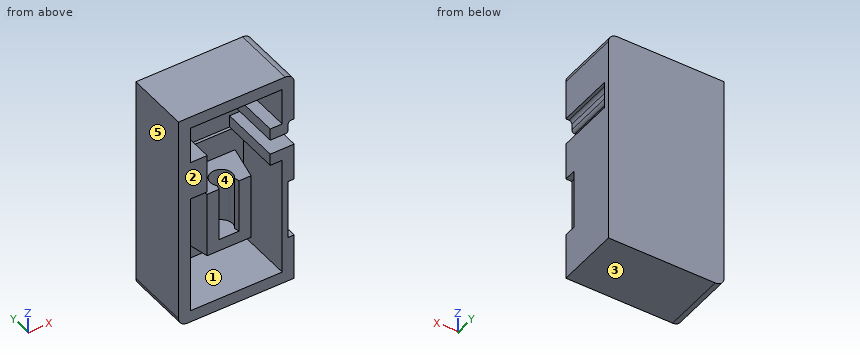
Autodesk Inventor part; units mm, degrees
ref_plane "YZ Plane" through (0, 0, 0) normal (1, 0, 0) x (0, 1, 0)
ref_plane "XZ Plane" through (0, 0, 0) normal (0, 1, 0) x (-1, 0, 0)
ref_plane "XY Plane" through (0, 0, 0) normal (0, 0, 1) x (1, 0, 0)
sketch "Sketch1" plane through (0, 0, 0) normal (0, 1, 0) x (-1, 0, 0)
  line L0 (0, 0) -> (24.5364, 0)
  line L1 (24.5364, 0) -> (24.5364, -46.5582)
  line L2 (24.5364, -46.5582) -> (0, -46.5582)
  line L3 (0, -46.5582) -> (0, 0)
  dimension "d0" = 46.5582
  dimension "d1" = 24.5364
extrude "Extrusion1" add sketch "Sketch1" along normal blind 13.5382
sketch "Sketch2" plane through (0, 0, 0) normal (0, -1, 0) x (1, 0, 0)
  point P0 (0, 0)
fillet "Fillet1" radius 1.905 1 edges at (-24.5364, 6.7691, -46.5582)
fillet "Fillet2" radius 1.905 1 edges at (0, 6.7691, 0)
sketch "Sketch3" plane through (0, 0, 0) normal (0, -1, 0) x (1, 0, 0)
  line L0 (-1.905, 0) -> (-24.5364, 0)
  arc A0 (0, -1.905) -> (-1.905, 0) centre (-1.905, -1.905) ccw
  line L1 (0, -46.5582) -> (0, -1.905)
  line L2 (-22.6314, -46.5582) -> (0, -46.5582)
  arc A1 (-24.5364, -44.6532) -> (-22.6314, -46.5582) centre (-22.6314, -44.6532) ccw
  line L3 (-24.5364, 0) -> (-24.5364, -44.6532)
  line L4 (-2.54, -2.54) -> (-21.9964, -2.54)
  line L5 (-21.9964, -44.0182) -> (-2.54, -44.0182)
  line L6 (0, -12.9032) -> (-5.08, -12.9032)
  line L7 (-5.08, -16.0782) -> (0, -16.0782)
  line L8 (-2.54, -44.0182) -> (-2.54, -18.6182)
  line L9 (-2.54, -10.3632) -> (-2.54, -2.54)
  line L10 (-5.08, -12.9032) -> (-5.08, -10.3632)
  line L11 (-5.08, -10.3632) -> (-2.54, -10.3632)
  line L12 (-5.08, -16.0782) -> (-5.08, -18.6182)
  line L13 (-5.08, -18.6182) -> (-2.54, -18.6182)
  line L14 (-21.9964, -10.3632) -> (-18.4404, -10.3632)
  line L15 (-18.4404, -10.3632) -> (-18.4404, -18.6182)
  line L16 (-18.4404, -18.6182) -> (-21.9964, -18.6182)
  line L17 (-21.9964, -2.54) -> (-21.9964, -10.3632)
  line L18 (-21.9964, -18.6182) -> (-21.9964, -44.0182)
  line L19 (0, -14.4907) -> (-5.2569, -14.4907) construction
  line L20 (-5.08, -11.6332) -> (-18.4404, -11.6332)
  line L21 (-5.08, -17.3482) -> (-18.4404, -17.3482)
  point P0 (0, 0)
  dimension "d7" = 2.54
  dimension "d9" = 2.54
  dimension "d11" = 3.175
  dimension "d13" = 5.08
  dimension "d14" = 2.54
  dimension "d15" = 2.54
  dimension "d16" = 2.54
  dimension "d17" = 2.54
  dimension "d20" = 2.54
  dimension "d21" = 6.096
  dimension "d22" = 2.54
  dimension "d37" = 32.0675
extrude "Extrusion2" cut sketch "Sketch3" against normal blind 12.2682 contours L1 L7 L12 L21 L15 L20 L10 L6 | L20 L15 L14 L17 L4 L9 L11 L10 | L12 L13 L8 L5 L18 L16 L15 L21
sketch "Sketch4" plane through (0, 12.2682, 0) normal (0, -1, 0) x (1, 0, 0)
  line L0 (-4.3434, -23.6982) -> (-17.0434, -23.6982)
  line L1 (-17.0434, -23.6982) -> (-17.0434, -35.1282)
  line L2 (-17.0434, -35.1282) -> (-4.3434, -35.1282)
  line L3 (-4.3434, -35.1282) -> (-4.3434, -23.6982)
  line L4 (-2.54, -44.0182) -> (-21.9964, -44.0182)
  line L5 (-2.54, -18.6182) -> (-2.54, -44.0182)
  line L6 (-10.6934, -23.6982) -> (-10.6934, -35.1282) construction
  line L7 (-24.5364, 0) -> (-24.5364, -44.6532) construction
  line L8 (-22.6314, -46.5582) -> (0, -46.5582) construction
  point P0 (0, 0)
  dimension "d23" = 13.843
  dimension "d24" = 12.7
  dimension "d25" = 11.43
  dimension "d26" = 22.86
extrude "Extrusion3" add sketch "Sketch4" along normal up to surface (12.2682 mm away)
sketch "Sketch5" plane through (-4.3434, 12.2682, -35.1282) normal (0, 0, -1) x (-1, 0, 0)
  line L0 (0, 0) -> (0, -12.2682)
  line L1 (12.7, 0) -> (12.7, -12.2682)
  line L2 (12.7, -12.2682) -> (0, -12.2682)
  arc A0 (8.2396, -6.5778) -> (4.4604, -6.5778) centre (6.35, -5.1816) ccw
  line L3 (6.35, -12.2682) -> (6.35, 0) construction
  line L4 (17.653, 0) -> (-1.8034, 0) construction
  line L5 (8.2396, -6.5778) -> (8.4707, -7.62)
  line L6 (8.4707, -7.62) -> (11.0107, -7.62)
  line L7 (11.0107, -7.62) -> (12.7, 0)
  line L8 (4.4604, -6.5778) -> (4.2293, -7.62)
  line L9 (4.2293, -7.62) -> (1.6893, -7.62)
  line L10 (1.6893, -7.62) -> (0, 0)
  point P0 (-4.3434, -12.2682)
  dimension "d29" = 7.0866
  dimension "d30" = 4.699
  dimension "d32" = 7.62
  dimension "d33" = 2.54
  dimension "d36" = 25
extrude "Extrusion4" cut sketch "Sketch5" against normal up to surface (11.43 mm away)
sketch "Sketch6" plane through (0, 12.2682, 0) normal (0, -1, 0) x (1, 0, 0)
  line L0 (-5.08, -10.3632) -> (-5.08, -12.9032)
  line L1 (-5.08, -16.0782) -> (-5.08, -18.6182)
  line L2 (-18.4404, -18.6182) -> (-18.4404, -10.3632)
  line L3 (0, -12.9032) -> (0, -16.0782)
  line L4 (0, -16.0782) -> (-5.08, -16.0782)
  line L5 (-5.08, -12.9032) -> (0, -12.9032)
  line L6 (-5.08, -10.3632) -> (-18.4404, -10.3632)
  line L7 (-18.4404, -18.6182) -> (-5.08, -18.6182)
  line L8 (-1.27, -12.9032) -> (-1.27, -16.0782)
  point P0 (0, 0)
  dimension "d46" = 1.27
extrude "Extrusion5" cut sketch "Sketch6" against normal blind 0.635
sketch "Sketch7" plane through (0, 0, 0) normal (0, -1, 0) x (1, 0, 0)
  line L0 (0, -12.9032) -> (0, -1.905)
  line L1 (0, -1.905) -> (0, -46.5582)
  line L2 (0, -10.3632) -> (-0.635, -10.3632)
  line L3 (-1.27, -10.9982) -> (-1.27, -12.2682)
  arc A0 (-0.635, -10.3632) -> (-1.27, -10.9982) centre (-0.635, -10.9982) ccw
  line L4 (-1.905, -12.9032) -> (-5.08, -12.9032)
  line L5 (-5.08, -10.3632) -> (-5.08, -12.9032)
  arc A1 (-1.905, -12.9032) -> (-1.27, -12.2682) centre (-1.905, -12.2682) ccw
  line L6 (0, -10.3632) -> (0, -12.9032)
  line L7 (0, -12.9032) -> (-1.905, -12.9032)
  line L8 (-5.08, -12.9032) -> (0, -12.9032)
  point P0 (0, 0)
  point P1 (-1.27, -10.3632)
  point P2 (-1.27, -12.9032)
  dimension "d40" = 1.27
  dimension "d41" = 2.54
  dimension "d42" = 0.635
  dimension "d43" = 0.635
extrude "Extrusion7" add sketch "Sketch6" against normal blind 0.635 contours L5 L3 L4 L8
extrude "Extrusion8" cut sketch "Sketch7" against normal up to surface (12.2682 mm away)
sketch "Sketch8" plane through (0, 0, -46.5582) normal (1, 0, 0) x (0, 0, -1)
  line L0 (-36.195, 0) -> (-36.195, 12.2682)
  line L1 (-30.48, 12.2682) -> (-36.195, 12.2682)
  line L2 (-30.48, 12.2682) -> (-30.48, 0)
  line L3 (0, 0) -> (-30.48, 0)
  line L4 (0, 0) -> (0, 13.5382)
  line L5 (-44.6532, 13.5382) -> (0, 13.5382)
  line L6 (-44.6532, 0) -> (-44.6532, 13.5382)
  line L7 (-36.195, 0) -> (-44.6532, 0)
  line L8 (-22.5397, 0) -> (-22.5397, 2.54)
  line L9 (-22.5397, 2.54) -> (-9.8397, 2.54)
  line L10 (-9.8397, 2.54) -> (-9.8397, 0)
  point P0 (-46.5582, 0)
  dimension "d51" = 2.54
  dimension "d52" = 12.7
extrude "Extrusion9" cut sketch "Sketch8" against normal blind 1.27 contours L8 L9 L10 L3
sketch "Sketch9" plane through (-4.3434, 12.2682, -35.1282) normal (0, 0, -1) x (-1, 0, 0)
  line L0 (12.7, 0) -> (11.0107, -7.62)
  line L1 (11.0107, -7.62) -> (8.4707, -7.62)
  line L2 (8.4707, -7.62) -> (8.2396, -6.5778)
  arc A0 (8.2396, -6.5778) -> (4.4604, -6.5778) centre (6.35, -5.1816) ccw
  line L3 (4.4604, -6.5778) -> (4.2293, -7.62)
  line L4 (4.2293, -7.62) -> (1.6893, -7.62)
  line L5 (1.6893, -7.62) -> (0, 0)
  line L6 (12.7, 0) -> (0, 0)
  line L7 (1.6893, -7.62) -> (11.0107, -7.62)
  line L8 (4.2293, -7.62) -> (1.6893, -7.62)
  point P0 (-4.3434, -12.2682)
extrude "Extrusion10" add sketch "Sketch9" along normal blind 2.54
equation "\"d27\" = d2"
equation "\"d34\" = d2"
properties part number "Negative CAp"
Read the model definition and answer for the solid it produces. Units are mm, in the model's axes. Face numbers are marked on the shaded views. A direction names the side the tool comes from. Give positions to 0.01 mm unless a question says otherwise; leave off trailing zeros. Write each loop counter-clockwise with the first axis right and the second up, starting at its lowest first coordinate (ties: lowest second). Pieces come first, ordered by that corner, then holes. Notation, with made-up numbers: (86, 74) - (102, 74) arc R32 ccw to (102, 105) - close; hole circle Ø6 at (17.25, 3). An arc over 180 degrees is marked (long way). Answer in a Markdown table with one row per item. Add a question column.
Item 1: Section C-C, the plane z = -30.5 is taken. Write down the section's boundary in (x, y), and give its area (3 significant figures).
Item 2: Find the intervals of material crossed by L1, parallel to Z at x = -10.5, y = 10.5; L2, parallel to Z at x = -11.25, y = 6.5; L3, parallel to Z at x = -3.25, y = 10.5, in increasing order.
Item 3: A tool of negligible diameter and unlimited length cuts with its end or side. For the marked faces 1 and 2, from which of +Z, -Z, +X, -X, +Y, -Y can it reach the whole face along a straight path? Write none if from no direction.
Item 4: Determine the mould class of the marked faces 3, 4 and 5 for opening direction Z: pulls with the +Z half, pulls with the -Z half, needs draft (parallel to the pull), parting line crosses it, or undercut.
Item 5: Flat-ended cylindrical pins translate along their axes: P1, Ø10.5, axis at x = -12.5, z = -34, coming from the -Y side; P2, Ø3, axis at y = 9.5, z = -14, coming from the +X side; P3, Ø1, axis at x = -17, z = -20, coming from the -Y side. Find the tip coordinate at first contact, or state that the pin passes through.
Item 6: Section B-B, the plane y = 3.5 is taken. Write down the section's boundary in (x, z) (3 decimals).
Item 7: Section A-A, the plane x = -7.75 is taken. Write down the section's boundary in (y, z).
Recorded:
| question | item | result |
|---|---|---|
| 1 | outline | (-24.54, 0) - (-22, 0) - (-22, 12.27) - (-17.04, 12.27) - (-15.35, 4.65) - (-12.81, 4.65) - (-12.58, 5.69) arc R2.35 cw (long way) to (-8.8, 5.69) - (-8.57, 4.65) - (-6.03, 4.65) - (-4.34, 12.27) - (-2.54, 12.27) - (-2.54, 0) - (-1.27, 0) - (-1.27, 2.54) - (0, 2.54) - (0, 13.54) - (-24.54, 13.54) - close |
| 1 | area | 155 mm2 |
| 2 | L1 | z = -46.56 to -44.02, -37.67 to -23.7, -2.54 to 0 |
| 2 | L2 | z = -46.56 to -44.02, -37.67 to -35.13, -2.54 to 0 |
| 2 | L3 | z = -46.56 to -44.02, -18.62 to -16.08, -12.9 to -10.36, -2.54 to 0 |
| 3 | face 1 | -Y |
| 3 | face 2 | +Z, -Z, +X, -X, -Y |
| 4 | face 3 | pulls with the -Z half |
| 4 | face 4 | undercut |
| 4 | face 5 | needs draft |
| 5 | P1 | stops at y = 4.65 |
| 5 | P2 | stops at x = -1.31 |
| 5 | P3 | stops at y = 12.27 |
| 6 | outline | (-24.536, -44.653) arc R1.905 ccw to (-22.631, -46.558) - (0, -46.558) - (0, -16.078) - (-5.08, -16.078) - (-5.08, -18.618) - (-2.54, -18.618) - (-2.54, -44.018) - (-21.996, -44.018) - (-21.996, -18.618) - (-18.44, -18.618) - (-18.44, -10.363) - (-21.996, -10.363) - (-21.996, -2.54) - (-2.54, -2.54) - (-2.54, -10.363) - (-5.08, -10.363) - (-5.08, -12.903) - (-1.905, -12.903) arc R0.635 ccw to (-1.27, -12.268) - (-1.27, -10.998) arc R0.635 cw to (-0.635, -10.363) - (0, -10.363) - (0, -1.905) arc R1.905 ccw to (-1.905, 0) - (-24.536, 0) - close |
| 7 | outline | (0, -46.56) - (13.54, -46.56) - (13.54, 0) - (0, 0) - (0, -2.54) - (12.27, -2.54) - (12.27, -10.36) - (12.9, -10.36) - (12.9, -18.62) - (12.27, -18.62) - (12.27, -23.7) - (4.65, -23.7) - (4.65, -37.67) - (12.27, -37.67) - (12.27, -44.02) - (0, -44.02) - close |
